```python
from build123d import *

# Parameters (mm, degrees)
BOSS_EXTRU_1_DEPTH           = 2
CONG_3_R                     = 1
D_GAGEMENT_M2_51_D           = 2.9
D_GAGEMENT_M2_51_CSINK_D     = 2.95
D_GAGEMENT_M2_51_CSINK_ANGLE = 90


with BuildPart() as part:
    # Esquisse1 → Boss.-Extru.1 (new body)
    with BuildSketch(Plane.XY):
        Polygon((-9.5, 19), (9.5, 19), (9.5, 6), (7.5, 6), (7.5, 0), (-7.5, 0), (-7.5, 6), (-9.5, 6), align=None)
    extrude(amount=BOSS_EXTRU_1_DEPTH)

    # Congé3
    cong_3_edges = [part.edges().sort_by_distance(p)[0] for p in [
        (9.5, 19, 1),
        (9.5, 6, 1),
        (7.5, 6, 1),
        (7.5, 0, 1),
        (-7.5, 0, 1),
        (-7.5, 6, 1),
        (-9.5, 6, 1),
        (-9.5, 19, 1),
    ]]
    fillet(cong_3_edges, radius=CONG_3_R - 0.0001)  # a hair under: the kernel refuses the full size

    # Dégagement M2.51 (through all)
    with Locations(Plane(origin=(-6.8, 16.3, 2), x_dir=(1, 0, 0), z_dir=(0, 0, 1))):
        with Locations((0, 0), (13.6, 0)):
            CounterSinkHole(D_GAGEMENT_M2_51_D / 2, D_GAGEMENT_M2_51_CSINK_D / 2, counter_sink_angle=D_GAGEMENT_M2_51_CSINK_ANGLE)


solid = part.part
```
Source: CAD feature listing. Evaluate the final solid. Frame: model axes, mm. A direction names the side the tool comes from. Coordinates: 2 decimals unless noted, no trailing zeros. Write each loop counter-clockwise with the first axis right and the second up, starting at its lowest first coordinate (ties: lowest second). Pieces come first, ordered by that corner, then holes. Notation, with made-up numbers: (69.5, 45) - (87.5, 45) arc R30 cw to (87.5, 72) - close; hole circle Ø8 at (32, -29). An arc over 180 degrees is marked (long way). Answer as a JSON object with one key per item and string values.
Q1. Section query C-C, the plane y = 4.25. Output: boundary loops of the cut face in (x, z).
Ans:
{"outline": "(-7.5, 0) - (7.5, 0) - (7.5, 2) - (-7.5, 2) - close"}
Q2. Set-up query: faces 5 (the flat face through (0, 10, 0)), 6 (the flat face through (-7.5, 3, 1)), 7 (the flat face through (7.5, 3, 1)). Return all of +Z, -Z, +X, -X, +Y, -Y with unobstructed straight access to the full face (end or side cutting, diameter ignored); none if empty.
Ans:
{"face 5": "-Z, +X, -X, +Y, -Y", "face 6": "+Z, -Z, -X, -Y", "face 7": "+Z, -Z, +X, -Y"}
Q3. Material intervals for line 1 (X direction, y = 16.3, z = 1.05); line 2 (X direction, y = 17.5, z = 1.15); line 3 (X direction, y = 1.25, z = 0.45), sorted ascending. Write a range as [from, to].
Ans:
{"line 1": "x = [-9.5, -8.25], [-5.35, 5.35], [8.25, 9.5]", "line 2": "x = [-9.5, -7.61], [-5.99, 5.99], [7.61, 9.5]", "line 3": "x = [-7.5, 7.5]"}
Q4. Section query B-B, the plane x = -6.8. Output: boundary loops of the cut face in (y, z) (3 decimals).
Ans:
{"outline": "(0.046, 0) - (14.85, 0) - (14.85, 1.975) - (14.825, 2) - (0.046, 2) - close; (17.75, 0) - (19, 0) - (19, 2) - (17.775, 2) - (17.75, 1.975) - close"}
Q5. Section query A-A, the plane z = 1.35. State how many separate pieces and enclosed holes the cut face has, plus the area to 3 significant figures.
Ans:
{"separate pieces": "1", "enclosed holes": "2", "area": "323 mm2"}
Q6. First-contact query: pin 1 Ø3 at (x, y) = (5, 10) entering from -Z; pin 2 Ø1 at (y, z) = (3.5, 1) entering from -X. Flat tips, straight axial feed; report the tip coordinate or a pass-through.
Ans:
{"pin 1": "stops at z = 0", "pin 2": "stops at x = -7.5"}
Q7. Draft query along Y for faces 1 (the cylindrical face through (5.42, 16.74, 0.97)), 2 (the flat face through (0, 0, 1)), 3 (the cylindrical face through (-5.65, 15.42, 0.97)), 4 (the flat face through (-9.5, 12, 1)). Return one class per face: released by +Y, released by -Y, zero draft, split by the parting line, or undercut.
Ans:
{"face 1": "undercut", "face 2": "released by -Y", "face 3": "undercut", "face 4": "zero draft"}
